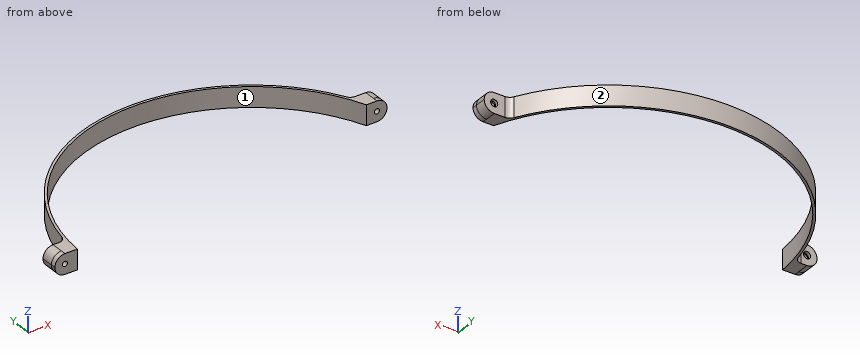
```python
from build123d import *

# Parameters (mm, degrees)
RESSALTO_EXTRUS_O6_DEPTH  = 20
FILETE4_R                 = 10
FILETE5_R                 = 10
RESSALTO_EXTRUS_O14_DEPTH = 17
RESSALTO_EXTRUS_O15_DEPTH = 16
FILETE6_R                 = 7
FILETE7_R                 = 7
ESBO_O25_R                = 2.5
CORTE_EXTRUS_O1_DEPTH     = 16
ESBO_O27_R                = 2.5
CORTE_EXTRUS_O2_DEPTH     = 18
ESBO_O28_R                = 3.55
CORTE_EXTRUS_O3_DEPTH     = 3.1
ESBO_O29_R                = 2.5
CORTE_EXTRUS_O4_DEPTH     = 22.1
ESBO_O30_R                = 3.55
CORTE_EXTRUS_O5_DEPTH     = 3.1


# Some blends are built 0.0001 mm under size
with BuildPart() as part:
    # Esboço2 → Ressalto-extrusão6 (new body)
    with BuildSketch(Plane.XY):
        with BuildLine():
            Line((157.082780724, 65), (177.082780724, 65))
            Line((177.082780724, 65), (177.082780724, 60))
            Line((177.082780724, 60), (156.38494173, 60))
            ThreePointArc((156.38494173, 60), (-25.578272063, 165.535500719), (-167.201226072, 10))
            Line((-167.201226072, 10), (-189.705627485, 10))
            Line((-189.705627485, 10), (-189.705627485, 15))
            Line((-189.705627485, 15), (-169.336942219, 15))
            ThreePointArc((-169.336942219, 15), (-25.739874096, 168.040051421), (157.082780724, 65))
        make_face()
    extrude(amount=RESSALTO_EXTRUS_O6_DEPTH)

    # Filete4
    filete4_edges = [part.edges().sort_by_distance(p)[0] for p in [
        (177.082780724, 62.5, 0),
        (177.082780724, 62.5, 20),
    ]]
    fillet(filete4_edges, radius=FILETE4_R - 0.0001)  # a hair under: the kernel refuses the full size

    # Filete5
    filete5_edges = [part.edges().sort_by_distance(p)[0] for p in [
        (-189.705627485, 12.5, 0),
        (-189.705627485, 12.5, 20),
    ]]
    fillet(filete5_edges, radius=FILETE5_R - 0.0001)  # a hair under: the kernel refuses the full size

    # Esboço20 → Ressalto-extrusão14 (add)
    with BuildSketch(Plane.XZ.offset(-10)):
        with BuildLine():
            Line((-167.201226072, 20), (-167.201226072, 0))
            Line((-167.201226072, 0), (-179.705627485, 0))
            ThreePointArc((-179.705627485, 0), (-186.776695297, 2.928932188), (-189.705627485, 10))
            ThreePointArc((-189.705627485, 10), (-186.776695297, 17.071067812), (-179.705627485, 20))
            Line((-179.705627485, 20), (-167.201226072, 20))
        make_face()
    extrude(amount=-RESSALTO_EXTRUS_O14_DEPTH)

    # Esboço21 → Ressalto-extrusão15 (add)
    with BuildSketch(Plane.XZ.offset(-60)):
        with BuildLine():
            Line((156.38494173, 20), (156.38494173, 0))
            Line((156.38494173, 0), (167.082780724, 0))
            ThreePointArc((167.082780724, 0), (174.153848536, 2.928932188), (177.082780724, 10))
            ThreePointArc((177.082780724, 10), (174.153848536, 17.071067812), (167.082780724, 20))
            Line((167.082780724, 20), (156.38494173, 20))
        make_face()
    extrude(amount=-RESSALTO_EXTRUS_O15_DEPTH)

    # Filete6
    # the kernel refuses this fillet: 7 mm, written as the material it adds along each edge
    with BuildSketch(Plane(origin=(156.38494173, 66.66145813, 20), x_dir=(0, 1, 0), z_dir=(0, 0, -1))) as filete6_piece_1:
        with BuildLine():
            CenterArc((16.33834975, -0.051861764), FILETE6_R, 179.575501806, 62.459929256)
            Line((13.055871472, -6.234525943), (12.990221907, -6.358179227))
            ThreePointArc((12.990221907, -6.358179227), (6.533962206, -3.104642795), (-0.054897671, -0.128787599))
            Line((-0.054897671, -0.128787599), (0, 0.14))
            ThreePointArc((0, 0.14), (4.669270935, 0.14), (9.198545713, 0.001037235))
            Line((9.198545713, 0.001037235), (9.33854187, 0))
        make_face()
    extrude(amount=20)

    # Filete7
    filete7_edges = [part.edges().sort_by_distance(p)[0] for p in [
        (-167.842187784, 27, 10),
    ]]
    fillet(filete7_edges, radius=FILETE7_R)

    # Esboço25 → Corte-extrusão1 (cut)
    with BuildSketch(Plane.XZ.offset(-10)):
        with Locations((-179.705627485, 10)):
            Circle(ESBO_O25_R)
    extrude(amount=-CORTE_EXTRUS_O1_DEPTH, mode=Mode.SUBTRACT)

    # Esboço27 → Corte-extrusão2 (cut)
    with BuildSketch(Plane.XZ.offset(-10)):
        with Locations((-179.705627485, 10)):
            Circle(ESBO_O27_R)
    extrude(amount=-CORTE_EXTRUS_O2_DEPTH, mode=Mode.SUBTRACT)

    # Esboço28 → Corte-extrusão3 (cut)
    with BuildSketch(Plane(origin=(0, 27, 0), x_dir=(1, 0, 0), z_dir=(0, 1, 0))):
        with Locations(Location((-179.705627485, -10, 0), (0, 0, 180))):
            Circle(ESBO_O28_R)
    extrude(amount=-CORTE_EXTRUS_O3_DEPTH, mode=Mode.SUBTRACT)

    # Esboço29 → Corte-extrusão4 (cut)
    with BuildSketch(Plane.XZ.offset(-60)):
        with Locations(Location((167.082780724, 10, 0), (0, 0, 270))):
            Circle(ESBO_O29_R)
    extrude(amount=-CORTE_EXTRUS_O4_DEPTH, mode=Mode.SUBTRACT)

    # Esboço30 → Corte-extrusão5 (cut)
    with BuildSketch(Plane(origin=(0, 76, 0), x_dir=(1, 0, 0), z_dir=(0, 1, 0))):
        with Locations(Location((167.082780724, -10, 0), (0, 0, 270))):
            Circle(ESBO_O30_R)
    extrude(amount=-CORTE_EXTRUS_O5_DEPTH, mode=Mode.SUBTRACT)


solid = part.part
```
Check sheet for the modelled part. Datum: model origin and axes. Units: mm. Face numbers are marked on the shaded views. Give positions to 0.01 mm unless a question says otherwise; leave off trailing zeros. Order: outer loops, then holes, each group sorted by start corner. A loop starts at its lowest first (then second) coordinate and runs counter-clockwise, first axis right, second up. Notation, with made-up numbers: M -3.5,31 L 35.5,31 A19 cw 35.5,41 Z; hole C 82.5,72 d5. An arc over 180 degrees is marked long. Answer in a Markdown table with one row per item. Add a question column.
Q1. Thickness scan on L1, parallel to X at y = 75, z = 10; L2, parallel to X at y = 70, z = 10; L3, parallel to Y at x = -0.5, z = 8. Record the ranges inside material, lowest first.
Q2. Sectioned sample at B-B, the plane x = 123. Record the boundary of the cut face in (y, z).
Q3. Sectioned sample at C-C, the plane x = -75. Record the boundary of the cut face in (y, z).
Q4. Gauge pin test, flat ends, axial feed: pin 1 Ø8 at (x, z) = (-185.5, 17.5) entering from +Y; pin 2 Ø6 at (x, z) = (-179.71, 10) entering from -Y; pin 3 Ø3 at (x, z) = (172.5, 14) entering from +Y; pin 4 Ø6.5 at (x, z) = (167.08, 10) entering from +Y. Record the tip position at first contact, or that the pin passes through.
Q5. Sectioned sample at A-A, the plane y = 123. Record the boundary of the cut face in (x, z), and give its area (3 significant figures).
Q6. Release check for a two-part mould opening along X. For the marked faces 1 and 2 record: released by +X, released by -X, zero draft, split by the parting line, or undercut.
Verdict:
| question | item | result |
|---|---|---|
| 1 | L1 | -152.56 to -149.77, 149.77 to 163.53, 170.63 to 177.08 |
| 1 | L2 | -154.92 to -152.17, 152.17 to 164.58, 169.58 to 177.08 |
| 1 | L3 | 167.5 to 170 |
| 2 | outline | M 113.7,0 L 117.35,0 L 117.35,20 L 113.7,20 Z |
| 3 | outline | M 149.77,0 L 152.56,0 L 152.56,20 L 149.77,20 Z |
| 4 | pin 1 | y = 27 |
| 4 | pin 2 | y = 10 |
| 4 | pin 3 | y = 76 |
| 4 | pin 4 | y = 72.9 |
| 5 | outline | M -117.35,0 L -113.7,0 L -113.7,20 L -117.35,20 Z; M 113.7,0 L 117.35,0 L 117.35,20 L 113.7,20 Z |
| 5 | area | 146 mm² |
| 6 | face 1 | undercut |
| 6 | face 2 | split by the parting line |
